Read the model definition and answer for the solid it produces. Units are mm, in the model's axes. Face numbers are marked on the shaded views. A direction names the side the tool comes from. Round coordinates to 2 decimals unless told otherwise and drop trailing zeros. Write each loop counter-clockwise with the first axis right and the second up, starting at its lowest first coordinate (ties: lowest second). Pieces come first, ordered by that corner, then holes. Notation, with made-up numbers: (62.25, -35.5) -> (69.25, -35.5) arc R23 cw to (69.25, -12.5) -> close; hole circle Ø2 at (77.5, 20.25). An arc over 180 degrees is marked (long way). Return JSON: item names as keys, results as strings.
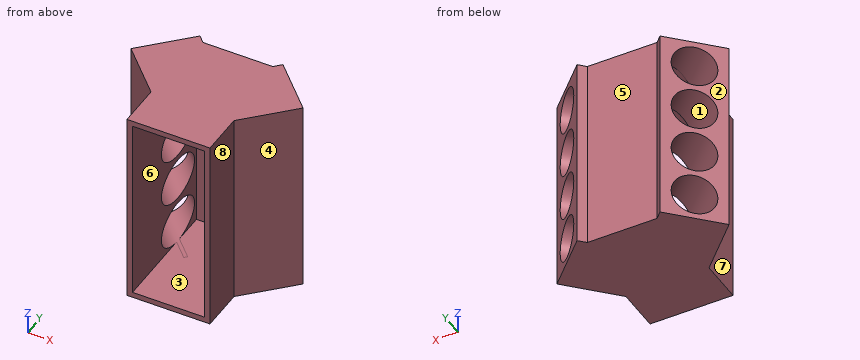
from build123d import *

# Parameters (mm, degrees)
SKETCH1_W           = 100
SKETCH1_H           = 358
BOSS_EXTRUDE1_DEPTH = 90
CHAMFER1_START      = -100
CHAMFER1_OUTLINE_W  = 113
CHAMFER1_OUTLINE_H  = 358
CHAMFER1_DEPTH      = 56.159379566
SKETCH3_W           = 358
SKETCH3_H           = 90
BOSS_EXTRUDE2_DEPTH = 53
SKETCH4_W           = 150
SKETCH4_H           = 358
BOSS_EXTRUDE3_DEPTH = 150
SKETCH5_W           = 78
SKETCH5_H           = 358
CUT_EXTRUDE2_DEPTH  = 12
CHAMFER3_SIZE       = 83
SKETCH6_W           = 124
SKETCH6_H           = 358
CUT_EXTRUDE3_DEPTH  = 12
CHAMFER4_SIZE       = 13
SKETCH7_R           = 38.5
CUT_EXTRUDE4_DEPTH  = 115
SKETCH8_R           = 38.5
CUT_EXTRUDE5_DEPTH  = 115
SKETCH9_W           = 130
SKETCH9_H           = 338
CUT_EXTRUDE6_DEPTH  = 210


with BuildPart() as part:
    # Sketch1 → Boss-Extrude1 (new body)
    with BuildSketch(Plane(origin=(0, 0, 0), x_dir=(1, 0, 0), z_dir=(0, 1, 0))):
        Rectangle(SKETCH1_W, SKETCH1_H)
    extrude(amount=BOSS_EXTRUDE1_DEPTH)

    # Chamfer1: read off the stored shape, not the designer's step
    # Chamfer1 outline → Chamfer1 (cut)
    with BuildSketch(Plane(origin=(0, 0, 0), x_dir=(0.7071067811865474, 0.7071067811865477, 0), z_dir=(0.7071067811865476, -0.7071067811865476, 0)).offset(CHAMFER1_START)):
        with Locations((28.5, 0)):
            Rectangle(CHAMFER1_OUTLINE_W, CHAMFER1_OUTLINE_H)
    extrude(amount=CHAMFER1_DEPTH, mode=Mode.SUBTRACT)

    # Sketch3 → Boss-Extrude2 (add)
    with BuildSketch(Plane(origin=(50, 0, 0), x_dir=(0, 0, -1), z_dir=(1, 0, 0))):
        with Locations((0, 45)):
            Rectangle(SKETCH3_W, SKETCH3_H)
    extrude(amount=BOSS_EXTRUDE2_DEPTH)

    # Mirror2: part across plane


with BuildPart() as part_1:
    add(part.part)
    add(part.part.mirror(Plane(origin=(103, 0, 0), x_dir=(0, 0, 1), z_dir=(1, 0, 0))))

    # Sketch4 → Boss-Extrude3 (add)
    with BuildSketch(Plane.XZ):
        with Locations((103, 0)):
            Rectangle(SKETCH4_W, SKETCH4_H)
    extrude(amount=BOSS_EXTRUDE3_DEPTH)

    # Sketch5 → Cut-Extrude2 (cut)
    with BuildSketch(Plane.XZ):
        with Locations((-11, 0)):
            Rectangle(SKETCH5_W, SKETCH5_H)
        with Locations((217, 0)):
            Rectangle(SKETCH5_W, SKETCH5_H)
    extrude(amount=-CUT_EXTRUDE2_DEPTH, mode=Mode.SUBTRACT)

    # Chamfer3
    # the kernel refuses this chamfer: 83 mm, written as the material it adds along each edge
    with BuildSketch(Plane(origin=(178, 12, 179), x_dir=(0, -1, 0), z_dir=(0, 0, -1))) as chamfer3_piece_1_section:
        Polygon((CHAMFER3_SIZE, 0), (0, -CHAMFER3_SIZE), (0, 0), align=None)
    chamfer3_piece_1 = extrude(amount=358, mode=Mode.PRIVATE)
    chamfer3_piece_1 = split(chamfer3_piece_1, bisect_by=Plane(origin=(217, 51, 179), z_dir=(-0.7071067811865476, -0.7071067811865476, 0)), keep=Keep.TOP, mode=Mode.PRIVATE)
    add(chamfer3_piece_1)
    with BuildSketch(Plane(origin=(28, 12, 179), x_dir=(-1, 0, 0), z_dir=(0, 0, -1))) as chamfer3_piece_2_section:
        Polygon((CHAMFER3_SIZE, 0), (0, -CHAMFER3_SIZE), (0, 0), align=None)
    chamfer3_piece_2 = extrude(amount=358, mode=Mode.PRIVATE)
    chamfer3_piece_2 = split(chamfer3_piece_2, bisect_by=Plane(origin=(-11, 51, 179), z_dir=(0.7071067811865476, -0.7071067811865476, 0)), keep=Keep.TOP, mode=Mode.PRIVATE)
    add(chamfer3_piece_2)

    # Sketch6 → Cut-Extrude3 (cut)
    with BuildSketch(Plane(origin=(0, 90, 0), x_dir=(1, 0, 0), z_dir=(0, 1, 0))):
        with Locations((103, 0)):
            Rectangle(SKETCH6_W, SKETCH6_H)
    extrude(amount=-CUT_EXTRUDE3_DEPTH, mode=Mode.SUBTRACT)

    # Chamfer4
    # the kernel refuses this chamfer: 13 mm, written as the material it takes off along each edge
    with BuildSketch(Plane(origin=(165, 90, 212.431878844), x_dir=(0, -1, 0), z_dir=(0, 0, -1))) as chamfer4_piece_1_section:
        Polygon((CHAMFER4_SIZE, 0), (0, -CHAMFER4_SIZE), (0, 0), align=None)
    chamfer4_piece_1 = extrude(amount=424.863757687, mode=Mode.PRIVATE)
    chamfer4_piece_1 = split(chamfer4_piece_1, bisect_by=Plane(origin=(165, 78, 212.431878844), z_dir=(0, 1, 0)), keep=Keep.TOP, mode=Mode.PRIVATE)
    add(chamfer4_piece_1, mode=Mode.SUBTRACT)
    with BuildSketch(Plane(origin=(41, 90, -212.431878844), x_dir=(-1, 0, 0), z_dir=(0, 0, 1))) as chamfer4_piece_2_section:
        Polygon((CHAMFER4_SIZE, 0), (0, CHAMFER4_SIZE), (0, 0), align=None)
    chamfer4_piece_2 = extrude(amount=424.863757687, mode=Mode.PRIVATE)
    chamfer4_piece_2 = split(chamfer4_piece_2, bisect_by=Plane(origin=(41, 78, -212.431878844), z_dir=(0, 1, 0)), keep=Keep.TOP, mode=Mode.PRIVATE)
    add(chamfer4_piece_2, mode=Mode.SUBTRACT)

    # Sketch7 → Cut-Extrude4 (cut)
    with BuildSketch(Plane(origin=(-31, 31, 0), x_dir=(0, 0, 1), z_dir=(-0.7071067811865477, 0.7071067811865475, 0))):
        with Locations(Location((130.362769157, 26.516504294, 0), (0, 0, 270))):
            Circle(SKETCH7_R)
        with Locations(Location((43.362769157, 26.516504294, 0), (0, 0, 270))):
            Circle(SKETCH7_R)
        with Locations(Location((-43.637230843, 26.516504294, 0), (0, 0, 270))):
            Circle(SKETCH7_R)
        with Locations(Location((-130.637230843, 26.516504294, 0), (0, 0, 270))):
            Circle(SKETCH7_R)
    extrude(amount=-CUT_EXTRUDE4_DEPTH, mode=Mode.SUBTRACT)

    # Sketch8 → Cut-Extrude5 (cut)
    with BuildSketch(Plane(origin=(134, 134, 0), x_dir=(0, 0, -1), z_dir=(0.7071067811865477, 0.7071067811865475, 0))):
        with Locations(Location((-130.5, -119.14749263, 0), (0, 0, 90))):
            Circle(SKETCH8_R)
        with Locations(Location((-43.5, -119.14749263, 0), (0, 0, 90))):
            Circle(SKETCH8_R)
        with Locations(Location((43.5, -119.14749263, 0), (0, 0, 90))):
            Circle(SKETCH8_R)
        with Locations(Location((130.5, -119.14749263, 0), (0, 0, 90))):
            Circle(SKETCH8_R)
    extrude(amount=-CUT_EXTRUDE5_DEPTH, mode=Mode.SUBTRACT)

    # Sketch9 → Cut-Extrude6 (cut)
    with BuildSketch(Plane.XZ.offset(150)):
        with Locations((103, 0)):
            Rectangle(SKETCH9_W, SKETCH9_H)
    extrude(amount=-CUT_EXTRUDE6_DEPTH, mode=Mode.SUBTRACT)


solid = part_1.part
Item 1: Section C-C (z = 35) is taken. Give the vertices of the cut face in (x, y), then the cut area to 3 significant figures.
Worked answers:
{"outline": "(-52.5, 9.5) -> (28, -71) -> (28, -150) -> (38, -150) -> (38, -53.65) -> (-38.82, 23.18) -> close; (14.32, 76.32) -> (38, 52.65) -> (38, 60) -> (168, 60) -> (168, 52.6) -> (191.7, 76.3) -> (178, 90) -> (166, 78) -> (40, 78) -> (28, 90) -> close; (168, -150) -> (178, -150) -> (178, -71) -> (258.5, 9.5) -> (244.8, 23.2) -> (168, -53.6) -> close", "area": "9,330 mm2"}
Item 2: Straight lines are drawn through the part: L1, parallel to Z at x = 80.5, y = 33; L2, parallel to Y at x = 100, z = 73.5; L3, parallel to X at y = -111.5, z = 76. For each, find the intervals that lie inside material, in ascending order. Write a range as [from, to].
Worked answers:
{"L1": "z = [-179, -169], [169, 179]", "L2": "y = [60, 78]", "L3": "x = [28, 38], [168, 178]"}
Item 3: For a pull along X with two mould halves and no side action, classify the marked faces 1, 2, 3 and 4 as released by +X, released by -X, zero draft, split by the parting line, or undercut.
Worked answers:
{"face 1": "undercut", "face 2": "released by -X", "face 3": "undercut", "face 4": "released by +X"}
Item 4: Section A-A (y = -107) is taken. Give the vertices of the cut face in (x, z), then the cut area to 3 significant figures.
Worked answers:
{"outline": "(28, -179) -> (178, -179) -> (178, 179) -> (28, 179) -> close; hole (38, -169) -> (168, -169) -> (168, 169) -> (38, 169) -> close", "area": "9,760 mm2"}
Item 5: Section D-D (y = 39) is taken. State how many separate pieces and enclosed holes the cut face has, then the cut area to 3 significant figures.
Worked answers:
{"separate pieces": "8", "enclosed holes": "0", "area": "11,400 mm2"}
Item 6: A tool of negligible diameter and unlimited length cuts with its end or side. For the marked faces 5, 6, 7 and 8, from which of +Z, -Z, +X, -X, +Y, -Y can it reach the whole face along a straight path? Write none if from no direction.
Worked answers:
{"face 5": "+Z, -Z, +Y", "face 6": "-Y", "face 7": "+Z, -Z, -X, -Y", "face 8": "+Z, -Z, +X, -Y"}
Item 7: Flat-ended cylindrical pins translate along their axes: pin 1 (23.5 mm diameter, centred on y = -111, z = 30, fed in from -X); pin 2 (6 mm diameter, centred on x = 19.5, z = 79.5, fed in from +Y); pin 3 (1.5 mm diameter, centred on y = -28.5, z = -129, fed in from +X). Find the tip coordinate at first contact, or state that the pin passes through.
Worked answers:
{"pin 1": "stops at x = 28", "pin 2": "stops at y = 84.5", "pin 3": "stops at x = 221.25"}
Item 8: Section B-B (z = 145.5) is taken. Give the vertices of the cut face in (x, y), then the cut area to 3 significant figures.
Worked answers:
{"outline": "(-52.5, 9.5) -> (28, -71) -> (28, -150) -> (38, -150) -> (38, -50.56) -> (-37.28, 24.72) -> close; (12.78, 74.78) -> (38, 49.56) -> (38, 60) -> (168, 60) -> (168, 49.64) -> (193.18, 74.82) -> (178, 90) -> (166, 78) -> (40, 78) -> (28, 90) -> close; (168, -150) -> (178, -150) -> (178, -71) -> (258.5, 9.5) -> (243.32, 24.68) -> (168, -50.64) -> close", "area": "9,930 mm2"}
